Solid Edge part; units mm, degrees
sketch "Sketch1" plane through (0, 0, 0) normal (0, 0, 1) x (1, 0, 0)
  line L0 (75.9968, 0.2032) -> (0.2032, 0.2032)
  line L1 (0.2032, 0.2032) -> (0.2032, 9.4107)
  line L2 (0.2032, 9.4107) -> (-0.4318, 9.4107)
  line L3 (-0.4318, 9.4107) -> (-0.4318, 19.1643)
  line L4 (-0.4318, 19.1643) -> (0.2032, 19.1643)
  line L5 (0.2032, 19.1643) -> (0.2032, 28.3718)
  line L6 (0.2032, 28.3718) -> (75.9968, 28.3718)
  line L7 (75.9968, 28.3718) -> (75.9968, 0.2032)
extrude "Protrusion1" add sketch "Sketch1" against normal up to vertex (1.5875 mm away)
sketch "Sketch2" plane through (38.1, 28.3718, -0.7937) normal (0, 1, 0) x (1, 0, 0)
  line L0 (34.6376, 2.3812) -> (38.862, -1.8431)
  line L1 (38.862, -1.8431) -> (38.862, 2.3812)
  line L2 (38.862, 2.3812) -> (34.6376, 2.3812)
extrude "Cutout1" cut sketch "Sketch2" against normal up to next
sketch "Sketch3" plane through (36.9467, 14.2875, -1.5875) normal (0, 0, -1) x (1, 0, 0)
  line L0 (-27.4217, -4.8768) -> (-36.7435, -4.8768)
  line L1 (-36.7435, -4.8768) -> (-36.7435, 4.8768)
  line L2 (-36.7435, 4.8768) -> (-27.4217, 4.8768)
  line L3 (-27.4217, 4.8768) -> (-27.4217, -4.8768)
extrude "Protrusion2" add sketch "Sketch3" along normal up to vertex (2.4765 mm away)
sketch "Sketch4" plane through (37.7404, 14.2875, 0) normal (0, 0, 1) x (1, 0, 0)
  circle A0 centre (-31.3904, 0) radius 1.7272
extrude "Cutout2" cut sketch "Sketch4" against normal through all
sketch "Sketch5" plane through (37.7404, 14.2875, 0) normal (0, 0, 1) x (1, 0, 0)
  circle A0 centre (-31.3904, 0) radius 2.921
extrude "Cutout3" cut sketch "Sketch5" against normal blind 2.54
sketch "Sketch6" plane through (38.0579, 28.3718, -0.7937) normal (0, 1, 0) x (1, 0, 0)
  line L0 (33.5337, 3.9052) -> (30.5442, 0.7937)
  line L1 (30.5442, 0.7937) -> (30.5442, -0.7937)
  line L2 (30.5442, -0.7937) -> (37.8547, -0.7937)
  line L3 (37.8547, -0.7937) -> (34.4257, 2.6352)
  line L4 (34.4257, 2.6352) -> (37.5977, 2.6352)
  line L5 (37.5977, 2.6352) -> (37.5977, 3.9052)
  line L6 (37.5977, 3.9052) -> (33.5337, 3.9052)
extrude "Protrusion3" add sketch "Sketch6" against normal up to vertex (28.1686 mm away)
sketch "Sketch7" plane through (34.4027, 14.2875, -1.5875) normal (0, 0, -1) x (1, 0, 0)
  line L0 (-24.6237, 12.4968) -> (37.1889, 12.4968)
  line L1 (37.1889, 12.4968) -> (37.1889, 14.0843)
  line L2 (37.1889, 14.0843) -> (-24.6237, 14.0843)
  line L3 (-24.6237, 14.0843) -> (-24.6237, 12.4968)
extrude "Protrusion4" add sketch "Sketch7" along normal up to vertex (3.1115 mm away)
Geometry check sheet. Reference: the model listing, model coordinates, mm. A direction names the side the tool comes from. Give positions to 0.01 mm unless a question says otherwise; leave off trailing zeros. Loops run counter-clockwise (first coordinate to the right, second up) from the corner with the lowest first, then second, coordinate; pieces in that order, holes last.
(1) Release check for a two-part mould opening along X. For faces 1 (the flat face through (41, 1, -4.699)), 2 (the flat face through (-0.432, 14, -1)), 3 (the flat face through (35, 14, -1.588)) record: released by +X, released by -X, zero draft, split by the parting line, or undercut.
From the geometry:
face 1: zero draft
face 2: released by -X
face 3: undercut
(2) Set-up check for faces 4 (the flat face through (5, 19.164, -3)), 5 (the flat face through (4, 14, -4.064)), 6 (the flat face through (75.656, 14, -4)), 7 (the cylindrical face through (5.97, 17.184, -1.252)): record each of +Z, -Z, +X, -X, +Y, -Y from which the full face is reachable in a straight line by a thin tool's end or side.
From the geometry:
face 4: -Z, -X, +Y
face 5: -Z, -X, +Y, -Y
face 6: -Z, +X, +Y, -Y
face 7: +Z
(3) Section check A-A on x = 6.35. Record the cut outline in (y, z).
From the geometry:
outline: (0.2, -1.59) - (9.41, -1.59) - (9.41, -4.06) - (12.56, -4.06) - (12.56, -2.54) - (11.37, -2.54) - (11.37, 0) - (0.2, 0) - close; (16.01, -4.06) - (19.16, -4.06) - (19.16, -1.59) - (28.37, -1.59) - (28.37, 0) - (17.21, 0) - (17.21, -2.54) - (16.01, -2.54) - close
(4) Section check D-D on y = 22. Record the cut outline in (x, z).
From the geometry:
outline: (0.2, -1.59) - (68.6, -1.59) - (71.59, -4.7) - (75.66, -4.7) - (75.66, -3.43) - (72.48, -3.43) - (75.91, 0) - (0.2, 0) - close
(5) Section check B-B on y = 18.25. Record the cut outline in (x, z) (1 decimal), then the cut area to 3 significant figures.
From the geometry:
outline: (-0.4, -1.6) - (0.2, -1.6) - (0.2, -4.1) - (9.5, -4.1) - (9.5, -1.6) - (68.6, -1.6) - (71.6, -4.7) - (75.7, -4.7) - (75.7, -3.4) - (72.5, -3.4) - (75.9, 0) - (-0.4, 0) - close
area: 156 mm2
(6) Thickness scan on L1, parallel to X at y = 13.5, z = -2.25 (3 decimals); L2, parallel to Z at x = 52, y = 21.5; L3, parallel to Y at x = 6.35, z = -1.1. Record the ranges inside material, lowest first.
From the geometry:
L1: x = 0.203 to 3.537, 9.163 to 9.525, 69.239 to 73.663
L2: z = -1.59 to 0
L3: y = 0.2 to 11.37, 17.21 to 28.37
(7) Section check C-C on x = 65. Record the cut outline in (y, z).
From the geometry:
outline: (0.2, -4.7) - (1.79, -4.7) - (1.79, -1.59) - (28.37, -1.59) - (28.37, 0) - (0.2, 0) - close
(8) Depth check by flat-ended pin: pin 1 Ø7.5 at (x, y) = (5, 13.5) entering from -Z; pin 2 Ø2 at (x, y) = (6.35, 14.29) entering from -Z; pin 3 Ø2.5 at (x, z) = (7, -3) entering from -Y; pin 4 Ø3 at (x, y) = (5.5, 14.5) entering from +Z. Enter the tip coordinate at first touch or a pass-through.
From the geometry:
pin 1: stops at z = -4.06
pin 2: passes through
pin 3: stops at y = 9.41
pin 4: stops at z = -2.54
